The listing builds one solid part. Answer for the finished solid, in the listing's coordinates (mm). Face numbers are marked on the shaded views. A direction names the side the tool comes from. Round coordinates to 2 decimals unless told otherwise and drop trailing zeros. Order: outer loops, then holes, each group sorted by start corner. A loop starts at its lowest first (then second) coordinate and runs counter-clockwise, first axis right, second up. Notation, with made-up numbers: (67.25, 64) - (123.25, 64) arc R29 ccw to (123.25, 92) - close; hole circle Ø3 at (70, 63). An arc over 180 degrees is marked (long way). One line per item, written item: value. Start each with the question number.
1. Section C-C, the plane y = 12 is taken. Give the vertices of the cut face in (x, z), then the cut area to 3 significant figures.
2. A tool of negligible diameter and unlimited length cuts with its end or side. For the marked faces 4, 5 and 6, from which of +Z, -Z, +X, -X, +Y, -Y can it reach the whole face along a straight path? Write none if from no direction.
3. Flat-ended cylindrical pins translate along their axes: P1, Ø1.5, axis at x = 0, z = 5, coming from the +Y side; P2, Ø3, axis at y = 3, z = 3, coming from the +X side; P3, Ø6, axis at y = 7, z = 8, coming from the +X side. Find the tip coordinate at first contact, or state that the pin passes through.
4. Section B-B, the plane x = 0 is taken. Give the vertices of the cut face in (y, z).
5. Straight lines are drawn through the part: line 1 (Y direction, x = 0, z = 3); line 2 (Z direction, x = 0, y = 10.75); line 3 (X direction, y = 2, z = 3.5). For each, find the intervals that lie inside material, in ascending order.
6. Section D-D, the plane z = 7.5 is taken. Give the vertices of the cut face in (x, y), then the cut area to 3 significant figures.
7. For a pull along Y with two mould halves and no side action, classify the marked faces 1, 2 and 3 as released by +Y, released by -Y, zero draft, split by the parting line, or undercut.
8. Section A-A, the plane y = 0 is taken. Give the vertices of the cut face in (x, z).
from build123d import *

# Parameters (mm, degrees)
SKETCH_1_R          = 15
EXTRUDE_1_DEPTH     = 10
SKETCH_3_R          = 3
CUT_EXTRUDE_1_DEPTH = 24.452078799
SKETCH_2_R          = 2
CUT_EXTRUDE_2_DEPTH = 24.452078799
M3X0_5_1_REACH      = 35.912
M3X0_5_1_BORE_R     = 1.25
M3X0_5_2_REACH      = 35.912
M3X0_5_2_BORE_R     = 1.25


with BuildPart() as part:
    # ｽｹｯﾁ1 → ﾎﾞｽ - 押し出し1 (new body)
    with BuildSketch(Plane.XY):
        Circle(SKETCH_1_R)
    extrude(amount=EXTRUDE_1_DEPTH)

    # ｽｹｯﾁ3 → ｶｯﾄ - 押し出し1 (cut, through all)
    with BuildSketch(Plane(origin=(0, 0, 0), x_dir=(-1, 0, 0), z_dir=(0, 0, -1))):
        Circle(SKETCH_3_R)
    extrude(amount=-CUT_EXTRUDE_1_DEPTH, mode=Mode.SUBTRACT)

    # ｽｹｯﾁ2 → ｶｯﾄ - 押し出し2 (cut, through all)
    with BuildSketch(Plane.XY.offset(10)):
        with Locations((0, 7)):
            Circle(SKETCH_2_R)
    extrude(amount=-CUT_EXTRUDE_2_DEPTH, mode=Mode.SUBTRACT)

    # M3x0.5 ねじ穴1 bore (on position points) → M3x0.5 ねじ穴1 (cut, up to next)
    with BuildSketch(Plane(origin=(0, 15, 5), x_dir=(1, 0, 0), z_dir=(0, 1, 0)), mode=Mode.PRIVATE) as m3x0_5_1_sk1:
        Circle(M3X0_5_1_BORE_R)
    m3x0_5_1_tool1 = extrude(m3x0_5_1_sk1.sketch, amount=-M3X0_5_1_REACH, mode=Mode.PRIVATE) & part.part
    add(m3x0_5_1_tool1.solids().sort_by_distance((0, 15, 5))[0], mode=Mode.SUBTRACT)

    # M3x0.5 ねじ穴2 bore (on position points) → M3x0.5 ねじ穴2 (cut, up to next)
    with BuildSketch(Plane(origin=(0, -15, 5), x_dir=(-1, 0, 0), z_dir=(0, -1, 0)), mode=Mode.PRIVATE) as m3x0_5_2_sk1:
        Circle(M3X0_5_2_BORE_R)
    m3x0_5_2_tool1 = extrude(m3x0_5_2_sk1.sketch, amount=-M3X0_5_2_REACH, mode=Mode.PRIVATE) & part.part
    add(m3x0_5_2_tool1.solids().sort_by_distance((0, -15, 5))[0], mode=Mode.SUBTRACT)


solid = part.part
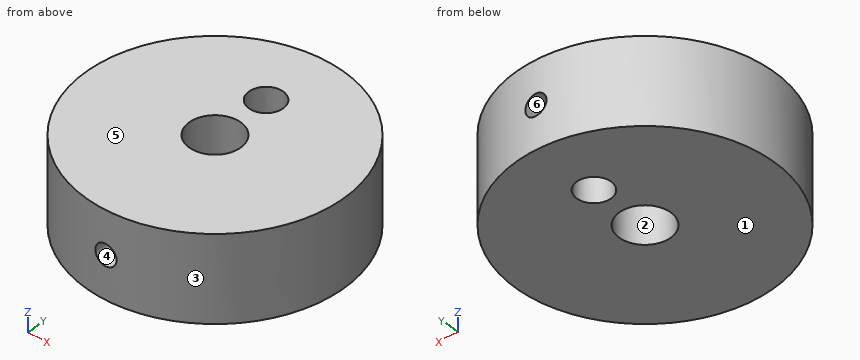
Answer list:
1. outline: (-9, 0) - (9, 0) - (9, 10) - (-9, 10) - close; hole circle Ø2.5 at (0, 5)
1. area: 175 mm²
2. face 4: -Y
2. face 5: +Z, +X, -X, +Y, -Y
2. face 6: +Y
3. P1: stops at y = 5.15
3. P2: stops at x = 14.92
3. P3: stops at x = 14.46
4. outline: (-15, 0) - (-3, 0) - (-3, 3.75) - (-15, 3.75) - close; (-15, 6.25) - (-3, 6.25) - (-3, 10) - (-15, 10) - close; (3, 0) - (5, 0) - (5, 10) - (3, 10) - close; (9, 0) - (15, 0) - (15, 3.75) - (9, 3.75) - close; (9, 6.25) - (15, 6.25) - (15, 10) - (9, 10) - close
5. line 1: y = -15 to -3, 3 to 5, 9 to 15
5. line 2: z = 0 to 3.75, 6.25 to 10
5. line 3: x = -14.87 to -2.24, 2.24 to 14.87
6. outline: circle Ø30 at (0, 0); hole circle Ø6 at (0, 0); hole circle Ø4 at (0, 7)
6. area: 666 mm²
7. face 1: zero draft
7. face 2: undercut
7. face 3: split by the parting line
8. outline: (-15, 0) - (-3, 0) - (-3, 10) - (-15, 10) - close; (3, 0) - (15, 0) - (15, 10) - (3, 10) - close
